from build123d import *

# Parameters (mm, degrees)
BOTTOMLAYER_DEPTH              = 4
MIDDLELAYER_DEPTH              = 2
FILLUPLAYER_START              = -2
FILLUPLAYER_DEPTH              = 2
TOPLAYER_DEPTH                 = 4
M3_CLEARANCE_HOLE1_D           = 3.4
M3_CLEARANCE_HOLE1_CSINK_D     = 6
M3_CLEARANCE_HOLE1_CSINK_ANGLE = 90
M2_5_CLEARANCE_HOLE1_D         = 2.9
CIRPATTERN1_COUNT              = 4
SKETCH30_R                     = 2.7
CUT_EXTRUDE1_DEPTH             = 3.4
CIRPATTERN2_COUNT              = 4


with BuildPart() as part:
    # Sketch3 → BottomLayer (new body)
    with BuildSketch(Plane.XY):
        with BuildLine():
            Line((0, 48), (48, 48))
            Line((48, 48), (48, 0))
            Line((48, 0), (46, 0))
            Line((46, 0), (46, 28))
            ThreePointArc((46, 28), (44.828427125, 30.828427125), (42, 32))
            Line((42, 32), (36, 32))
            ThreePointArc((36, 32), (33.171572875, 33.171572875), (32, 36))
            Line((32, 36), (32, 42))
            ThreePointArc((32, 42), (30.828427125, 44.828427125), (28, 46))
            Line((28, 46), (0, 46))
            Line((0, 46), (0, 48))
        make_face()
    bottomlayer = extrude(amount=BOTTOMLAYER_DEPTH)

    # Sketch6 → MiddleLayer (add)
    with BuildSketch(Plane.XY.offset(4)):
        with BuildLine():
            Line((0, 17.470562748), (0, 0))
            Line((0, 0), (17.470562748, 0))
            Line((17.470562748, 0), (17.470562748, 2.5))
            ThreePointArc((17.470562748, 2.5), (18.384008358, 7.092201188), (20.985281374, 10.985281374))
            Line((20.985281374, 10.985281374), (48, 38))
            Line((48, 38), (48, 48))
            Line((48, 48), (38, 48))
            Line((38, 48), (10.985281374, 20.985281374))
            ThreePointArc((10.985281374, 20.985281374), (7.092201188, 18.384008358), (2.5, 17.470562748))
            Line((2.5, 17.470562748), (0, 17.470562748))
        make_face()
    middlelayer = extrude(amount=MIDDLELAYER_DEPTH)

    # Sketch10 → FillUpLayer (add)
    with BuildSketch(Plane.XY.offset(6).offset(FILLUPLAYER_START)):
        with BuildLine():
            Line((48, 48), (0, 48))
            Line((0, 48), (0, 46))
            Line((0, 46), (28, 46))
            ThreePointArc((28, 46), (30.828427125, 44.828427125), (32, 42))
            Line((32, 42), (32, 36))
            ThreePointArc((32, 36), (33.171572875, 33.171572875), (36, 32))
            Line((36, 32), (42, 32))
            ThreePointArc((42, 32), (44.828427125, 30.828427125), (46, 28))
            Line((46, 28), (46, 0))
            Line((46, 0), (48, 0))
            Line((48, 0), (48, 48))
        make_face()
    filluplayer = extrude(amount=FILLUPLAYER_DEPTH)

    # Sketch11 → TopLayer (add)
    with BuildSketch(Plane.XY.offset(6)):
        with BuildLine():
            Line((48, 48), (0, 48))
            Line((0, 48), (0, 46))
            Line((0, 46), (28, 46))
            ThreePointArc((28, 46), (30.828427125, 44.828427125), (32, 42))
            Line((32, 42), (32, 36))
            ThreePointArc((32, 36), (33.171572875, 33.171572875), (36, 32))
            Line((36, 32), (42, 32))
            ThreePointArc((42, 32), (44.828427125, 30.828427125), (46, 28))
            Line((46, 28), (46, 0))
            Line((46, 0), (48, 0))
            Line((48, 0), (48, 48))
        make_face()
    toplayer = extrude(amount=TOPLAYER_DEPTH)

    # M3 Clearance Hole1 (through all)
    with Locations(Plane.XY.offset(10)):
        with Locations((41.525, 41.525)):
            m3_clearance_hole1 = CounterSinkHole(M3_CLEARANCE_HOLE1_D / 2, M3_CLEARANCE_HOLE1_CSINK_D / 2, counter_sink_angle=M3_CLEARANCE_HOLE1_CSINK_ANGLE)

    # M2.5 Clearance Hole1 (through all)
    with Locations(Plane.XY.offset(6)):
        with Locations((4.75, 4.75)):
            m2_5_clearance_hole1 = Hole(M2_5_CLEARANCE_HOLE1_D / 2)

    # CirPattern1: BottomLayer, MiddleLayer, FillUpLayer, TopLayer, M3 Clearance Hole1 ×4 about axis
    cirpattern1_axis = Axis((0, 0, 0), (0, 0, 1))
    add([bottomlayer.rotate(cirpattern1_axis, i * 360 / CIRPATTERN1_COUNT) for i in range(1, CIRPATTERN1_COUNT)])
    add([middlelayer.rotate(cirpattern1_axis, i * 360 / CIRPATTERN1_COUNT) for i in range(1, CIRPATTERN1_COUNT)])
    add([filluplayer.rotate(cirpattern1_axis, i * 360 / CIRPATTERN1_COUNT) for i in range(1, CIRPATTERN1_COUNT)])
    add([toplayer.rotate(cirpattern1_axis, i * 360 / CIRPATTERN1_COUNT) for i in range(1, CIRPATTERN1_COUNT)])
    add([m3_clearance_hole1.rotate(cirpattern1_axis, i * 360 / CIRPATTERN1_COUNT) for i in range(1, CIRPATTERN1_COUNT)], mode=Mode.SUBTRACT)

    # Sketch21 → Tap Drill M3 Side Plate (revolve, cut)
    with BuildSketch(Plane(origin=(48, 38.1, 5), x_dir=(0, 0, -1), z_dir=(0, 1, 0))):
        Polygon((0, 0), (0, 5.751075774), (1.25, 5), (1.25, 0), align=None)
    tap_drill_m3_side_plate = revolve(axis=Axis((54.35, 38.1, 5), (-1, 0, 0)), mode=Mode.SUBTRACT)

    # Camera Holes: M2.5 Clearance Hole1 across plane
    add(m2_5_clearance_hole1.mirror(Plane(origin=(0, 0, 0), x_dir=(0, 0, 1), z_dir=(-0.7071067811865476, -0.7071067811865476, 0))), mode=Mode.SUBTRACT)

    # Sketch27 → Tap Drill M3 Side Plate 2 (revolve, cut)
    with BuildSketch(Plane(origin=(38.1, 48, 5), x_dir=(0, 0, 1), z_dir=(1, 0, 0))):
        Polygon((0, 0), (0, 5.751075774), (1.25, 5), (1.25, 0), align=None)
    tap_drill_m3_side_plate_2 = revolve(axis=Axis((38.1, 54.35, 5), (0, -1, 0)), mode=Mode.SUBTRACT)

    # Sketch29 → Tap Drill M3 Rail (revolve, cut)
    with BuildSketch(Plane(origin=(45.5, 48, 5), x_dir=(0, 0, 1), z_dir=(1, 0, 0))):
        Polygon((0, 0), (0, 5.751075774), (1.25, 5), (1.25, 0), align=None)
    tap_drill_m3_rail = revolve(axis=Axis((45.5, 54.35, 5), (0, -1, 0)), mode=Mode.SUBTRACT)

    # SidePlate and Rail Holes 1: Tap Drill M3 Side Plate, Tap Drill M3 Side Plate 2, Tap Drill M3 Rail across plane
    add(tap_drill_m3_side_plate.mirror(Plane(origin=(0, 0, 0), x_dir=(0, 0, 1), z_dir=(1, 0, 0))), mode=Mode.SUBTRACT)
    add(tap_drill_m3_side_plate_2.mirror(Plane(origin=(0, 0, 0), x_dir=(0, 0, 1), z_dir=(1, 0, 0))), mode=Mode.SUBTRACT)
    add(tap_drill_m3_rail.mirror(Plane(origin=(0, 0, 0), x_dir=(0, 0, 1), z_dir=(1, 0, 0))), mode=Mode.SUBTRACT)

    # Side Plate and Rail Holes 2: Tap Drill M3 Side Plate, Tap Drill M3 Side Plate 2, Tap Drill M3 Rail across plane
    add(tap_drill_m3_side_plate.mirror(Plane.ZX), mode=Mode.SUBTRACT)
    add(tap_drill_m3_side_plate_2.mirror(Plane.ZX), mode=Mode.SUBTRACT)
    add(tap_drill_m3_rail.mirror(Plane.ZX), mode=Mode.SUBTRACT)

    # Side Plate and Rail Holes 2 copy 1 sketc → Side Plate and Rail Holes 2 copy 1 (revolve, cut)
    with BuildSketch(Plane(origin=(-48, -38.1, 5), x_dir=(0, 0, -1), z_dir=(0, -1, 0))):
        Polygon((0, 0), (0, 5.751075774), (1.25, 5), (1.25, 0), align=None)
    revolve(axis=Axis((-54.35, -38.1, 5), (1, 0, 0)), mode=Mode.SUBTRACT)

    # Side Plate and Rail Holes 2 copy 2 sketc → Side Plate and Rail Holes 2 copy 2 (revolve, cut)
    with BuildSketch(Plane(origin=(-38.1, -48, 5), x_dir=(0, 0, 1), z_dir=(-1, 0, 0))):
        Polygon((0, 0), (0, 5.751075774), (1.25, 5), (1.25, 0), align=None)
    revolve(axis=Axis((-38.1, -54.35, 5), (0, 1, 0)), mode=Mode.SUBTRACT)

    # Side Plate and Rail Holes 2 copy 3 sketc → Side Plate and Rail Holes 2 copy 3 (revolve, cut)
    with BuildSketch(Plane(origin=(-45.5, -48, 5), x_dir=(0, 0, 1), z_dir=(-1, 0, 0))):
        Polygon((0, 0), (0, 5.751075774), (1.25, 5), (1.25, 0), align=None)
    revolve(axis=Axis((-45.5, -54.35, 5), (0, 1, 0)), mode=Mode.SUBTRACT)

    # Sketch30 → Cut-Extrude1 (cut)
    with BuildSketch(Plane(origin=(0, 0, 0), x_dir=(-1, 0, 0), z_dir=(0, 0, -1))):
        with Locations((-41.525, 41.525)):
            Circle(SKETCH30_R)
    cut_extrude1 = extrude(amount=-CUT_EXTRUDE1_DEPTH, mode=Mode.SUBTRACT)

    # CirPattern2: Cut-Extrude1 ×4 about axis
    cirpattern2_axis = Axis((0, 0, 0), (0, 0, 1))
    for i in range(1, CIRPATTERN2_COUNT):
        add(cut_extrude1.rotate(cirpattern2_axis, i * 360 / CIRPATTERN2_COUNT), mode=Mode.SUBTRACT)


solid = part.part
Source: CAD feature listing. Evaluate the final solid. Frame: model axes, mm. A direction names the side the tool comes from. Coordinates: 2 decimals unless noted, no trailing zeros. Loops run counter-clockwise (first coordinate to the right, second up) from the corner with the lowest first, then second, coordinate; pieces in that order, holes last. Notation, with made-up numbers: (33, -18.75) - (41, -18.75) arc R28 cw to (41, 13.25) - close; hole circle Ø6 at (83, 66). An arc over 180 degrees is marked (long way). Return JSON: item names as keys, results as strings.
Q1. Access query for faces 4 (the flat face through (-35.8, -32.2, 10)), 5 (the cylindrical face through (44.222, 41.644, 1.676)), 6 (the conical face through (42.379, -38.232, 5.172)), 7 (the flat face through (-46, 0, 5)), 8 (the flat face through (-39, 32, 8)). Directions: +Z, -Z, +X, -X, +Y, -Y. A direction counts if a zero-diameter tool reaches every point of the face in a straight line with its end or side. Return the directions, or none.
Results:
{"face 4": "+Z, +X, -X, +Y, -Y", "face 5": "-Z", "face 6": "+X", "face 7": "+Z, -Z", "face 8": "+Z"}
Q2. Contact query for flat-ended pins moving along their axis: P1, Ø2.5, axis at x = -41.525, y = -41.525, coming from the +Z side; P2, Ø6, axis at x = -17, y = 6.5, coming from the -Z side; P3, Ø2.5, axis at x = 41, y = -40.5, coming from the -Z side; P4, Ø2, axis at x = 38.1, z = 5, coming from the -Y side. Output: stop coordinate, or through.
Results:
{"P1": "through", "P2": "z = 4", "P3": "z = 3.4", "P4": "y = -42.85"}
Q3. Material intervals for line 1 along X through (y, z) = (-46.9, 5); line 2 along Y through (x, z) = (-36, 6.75); line 3 along Y through (x, z) = (-23.5, 1.5), sorted ascending.
Results:
{"line 1": "-48 to -46.75, -44.25 to -39.35, -36.85 to 36.85, 39.35 to 44.25, 46.75 to 48", "line 2": "-48 to -32, 32 to 48", "line 3": "-48 to -46, 46 to 48"}
Q4. Section A-A, the plane y = 4.75. Return loops of the section in (x, z), plus the area to 3 significant figures.
Results:
{"outline": "(-48, 0) - (-46, 0) - (-46, 10) - (-48, 10) - close; (-17.68, 4) - (3.3, 4) - (3.3, 6) - (-17.68, 6) - close; (6.2, 4) - (17.68, 4) - (17.68, 6) - (6.2, 6) - close; (46, 0) - (48, 0) - (48, 10) - (46, 10) - close", "area": "105 mm2"}
Q5. Section B-B, the plane x = -4.75. Return loops of the section in (y, z).
Results:
{"outline": "(-48, 0) - (-46, 0) - (-46, 10) - (-48, 10) - close; (-17.68, 4) - (-6.2, 4) - (-6.2, 6) - (-17.68, 6) - close; (-3.3, 4) - (17.68, 4) - (17.68, 6) - (-3.3, 6) - close; (46, 0) - (48, 0) - (48, 10) - (46, 10) - close"}
Q6. Section D-D, the plane x = 34.5. Return loops of the section in (y, z).
Results:
{"outline": "(-48, 0) - (-32.29, 0) - (-32.29, 4) - (-24.5, 4) - (-24.5, 6) - (-32.29, 6) - (-32.29, 10) - (-48, 10) - close; (24.5, 4) - (32.29, 4) - (32.29, 0) - (48, 0) - (48, 10) - (32.29, 10) - (32.29, 6) - (24.5, 6) - close"}
Q7. Section C-C, the plane z = 2.25. Give the number of separate pieces and of enclosed holes in the cut face, plus the area to 3 significant figures.
Results:
{"separate pieces": "1", "enclosed holes": "5", "area": "1,460 mm2"}
Q8. Mould query, pull axis Y, two halves, no side actions, for faces 1 (the cylindrical face through (44.859, -30.797, 4.93)), 2 (the conical face through (45.285, -42.379, 4.972)), 3 (the conical face through (45.285, 42.379, 4.972)). Classes: released by +Y, released by -Y, zero draft, split by the parting line, or undercut.
Results:
{"face 1": "undercut", "face 2": "released by -Y", "face 3": "released by +Y"}
